For this review, take the finished solid that the model builds, in its own axes (mm). Face numbers are marked on the shaded views. A direction names the side the tool comes from. Round coordinates to 2 decimals unless told otherwise and drop trailing zeros. Write each loop counter-clockwise with the first axis right and the second up, starting at its lowest first coordinate (ties: lowest second). Pieces come first, ordered by that corner, then holes. Notation, with made-up numbers: (35.5, 36.25) - (51.5, 36.25) arc R17 cw to (51.5, 63.25) - close; hole circle Ø10 at (38, 33.5). An arc over 180 degrees is marked (long way). Answer in a Markdown table with one row per item. Add a question column.
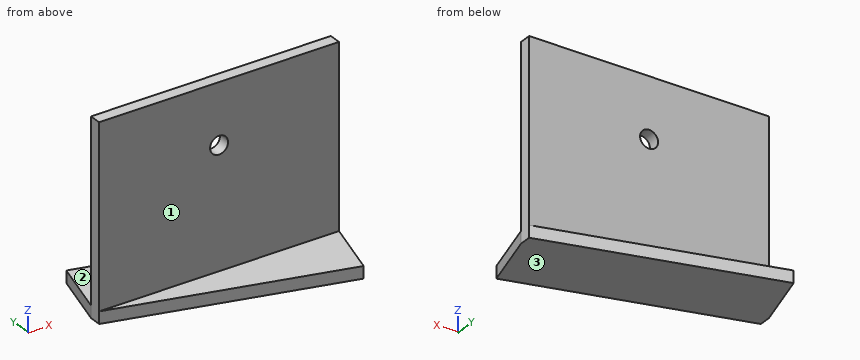
from build123d import *

# Parameters (mm, degrees)
SKETCH1_W           = 80
SKETCH1_H           = 60
BOSS_EXTRUDE1_DEPTH = 4
SKETCH2_R           = 3
CUT_EXTRUDE1_DEPTH  = 4
BOSS_EXTRUDE4_DEPTH = 4
SKETCH9_W           = 80
SKETCH9_H           = 4
BOSS_EXTRUDE5_DEPTH = 54
CUT_EXTRUDE5_DEPTH  = 54
CUT_EXTRUDE6_DEPTH  = 54
CUT_EXTRUDE7_DEPTH  = 54


with BuildPart() as part:
    # Sketch1 → Boss-Extrude1 (new body)
    with BuildSketch(Plane(origin=(0, 0, 0), x_dir=(1, 0, 0), z_dir=(0, 1, 0))):
        Rectangle(SKETCH1_W, SKETCH1_H)
    extrude(amount=BOSS_EXTRUDE1_DEPTH)

    # Sketch2 → Cut-Extrude1 (cut)
    with BuildSketch(Plane(origin=(0, 4, 0), x_dir=(1, 0, 0), z_dir=(0, 1, 0))):
        with Locations(Location((0, -10, 0), (0, 0, 270))):
            Circle(SKETCH2_R)
    extrude(amount=-CUT_EXTRUDE1_DEPTH, mode=Mode.SUBTRACT)



with BuildPart() as body_2:
    # Sketch8 → Boss-Extrude4 (new body)
    with BuildSketch(Plane(origin=(0, 0, -30), x_dir=(-1, 0, 0), z_dir=(0, 0, -1))):
        with BuildLine():
            Line((-40, 4), (37.274066103, 24.705523608))
            ThreePointArc((37.274066103, 24.705523608), (39.31558891, 14.442095378), (40, 4))
            Line((40, 4), (-40, 4))
        make_face()
    extrude(amount=BOSS_EXTRUDE4_DEPTH)


with BuildPart() as part_1:
    add(part.part)

    add(body_2.part)  # Boss-Extrude5 merges body 2
    # Sketch9 → Boss-Extrude5 (add)
    with BuildSketch(Plane.XZ.offset(-4)):
        with Locations((0, -32)):
            Rectangle(SKETCH9_W, SKETCH9_H)
    extrude(amount=BOSS_EXTRUDE5_DEPTH)

    # Sketch10 → Cut-Extrude5 (cut)
    with BuildSketch(Plane.XY.offset(-30)):
        Polygon((-40, 4), (-34.641016151, 24), (-48.042949513, 27.591037221), align=None)
    extrude(amount=-CUT_EXTRUDE5_DEPTH, mode=Mode.SUBTRACT)

    # Sketch11 → Cut-Extrude6 (cut)
    with BuildSketch(Plane.XY.offset(-30)):
        Polygon((40, 0), (26.602540378, -50), (60.406284328, -52.474789136), align=None)
    extrude(amount=-CUT_EXTRUDE6_DEPTH, mode=Mode.SUBTRACT)

    # Sketch12 → Cut-Extrude7 (cut)
    with BuildSketch(Plane.XY.offset(-30)):
        Polygon((-40, 0), (34.641016151, -20), (30.373618341, -54.228709826), (-68.422743557, -51.185946857), align=None)
    extrude(amount=-CUT_EXTRUDE7_DEPTH, mode=Mode.SUBTRACT)


solid = part_1.part
Q1. Tool access review of the marked faces 1, 2 and 3: name each direction out of +Z, -Z, +X, -X, +Y, -Y from which nothing blocks a thin tool from reaching the whole face with its end or side.
Q2. Add section D-D on z = -23. State the section outline as (x, y) points.
Q3. To check wall thickness, follow probe 1 along X at (y, z) = (2.25, 10); probe 2 along Y at (x, z) = (19, -7); probe 3 along Z at (x, y) = (-21, 18). State the ranges of each line that lie inside material, in increasing order.
Q4. Add section B-B on x = 0. State the section outline as (y, z) points, then the cut area to 3 significant figures.
Q5. Add section A-A on z = 10. State the section outline as (x, y) points.
Q6. Add section C-C on x = -16. State the section outline as (y, z) points.
Q7. Insertion check: pin 1 Ø10 at (x, z) = (-22.5, -24) entering from +Y; pin 2 Ø6 at (x, y) = (2.5, -12) entering from +Z. Each pin has a flat end and moves straight along its axis. Give the tip position at first contact, or say it passes through.
Answer sheet:
| question | item | result |
|---|---|---|
| 1 | face 1 | +Z, +X, -X, -Y |
| 1 | face 2 | +Z, +X, -X, +Y |
| 1 | face 3 | -Z, +X, -X, +Y, -Y |
| 2 | outline | (-40, 0) - (40, 0) - (40, 4) - (-40, 4) - close |
| 3 | probe 1 | x = -40 to -3, 3 to 40 |
| 3 | probe 2 | y = 0 to 4 |
| 3 | probe 3 | z = -34 to -30 |
| 4 | outline | (-10.72, -34) - (14.72, -34) - (14.72, -30) - (4, -30) - (4, 7) - (0, 7) - (0, -30) - (-10.72, -30) - close; (0, 13) - (4, 13) - (4, 30) - (0, 30) - close |
| 4 | area | 318 mm² |
| 5 | outline | (-40, 0) - (-3, 0) - (-3, 4) - (-40, 4) - close; (3, 0) - (40, 0) - (40, 4) - (3, 4) - close |
| 6 | outline | (-6.43, -34) - (19.01, -34) - (19.01, -30) - (4, -30) - (4, 30) - (0, 30) - (0, -30) - (-6.43, -30) - close |
| 7 | pin 1 | stops at y = 4 |
| 7 | pin 2 | stops at z = -30 |
